Here's how the part is built. I have some questions about the finished solid (model axes, mm). A direction names the side the tool comes from. Give positions to 0.01 mm unless a question says otherwise; leave off trailing zeros. Loops run counter-clockwise (first coordinate to the right, second up) from the corner with the lowest first, then second, coordinate; pieces in that order, holes last. Notation, with made-up numbers: (61.25, 48) -> (73.25, 48) arc R24 ccw to (73.25, 74) -> close; hole circle Ø4 at (-12, 21.5). An arc over 180 degrees is marked (long way). Answer in a Markdown table with one row per item. Add a question column.
Item 1: If we section it at B-B (y = 3): Write out the boundary of the cut face in (x, z) (3 decimals), then the cut area to 3 significant figures.
Item 2: If we section it at C-C (z = 0): Give the number of separate pieces and of enclosed holes in the cut face, then the cut area to 3 significant figures.
Item 3: Which directions (+Z, -Z, +X, -X, +Y, -Y) give clear straight access to the entire face, cutting with the end or side of a thin tool? Please do faces 4 (the face through (25, 11.684, 3)), 5 (the face through (-32, 1.905, 16)), 6 (the face through (-53.84, 15.62, 25.18)).
Item 4: We'd pull the mould along Z, two halves only. Please class faces 1 (the face through (-1, 8, 28.575)), 2 (the face through (25.44, 0.94, -19.16)), 3 (the face through (-53.837, 15.625, -25.173)): released by +Z, released by -Z, zero draft, split by the parting line, or undercut.
Item 5: If we section it at D-D (z = 20): Write out the boundary of the cut face in (x, y) (3 decimals).
Item 6: If I drill on line 1 (X direction, y = 6.25, z = -1); line 2 (Z direction, x = -31.75, y = 4) (3 decimals); line 3 (X direction, y = 1.75, z = -15), over which ranges is the centre line in solid material (lowest first)?
Item 7: For P1, Ø23, axis at x = -31.75, z = -15.875, coming from the -Y side; P2, Ø5, axis at x = 28, z = 16.5, coming from the -Y side (3 decimals); P3, Ø5, axis at x = 31.75, z = 0, coming from the -Y side, each with a flat end and sliding along its axis, tell me the tip position at first contact or that it passes through.
```python
from build123d import *

# Parameters (mm, degrees)
SKETCH1_W               = 114.3
SKETCH1_H               = 57.15
EXTRUDE1_DEPTH          = 15.875
CUT_EXTRUDE1_DEPTH      = 16.875
SKETCH4_R               = 15.5575
EXTRUDE7_DEPTH          = 4.191
SKETCH6_R               = 6.858
EXTRUDE8_DEPTH          = 4.191
CHAMFER1_SIZE           = 0.508
SKETCH7_R               = 7.112
CUT_EXTRUDE2_DEPTH      = 1.905
F_1_4_20_TAPPED_HOLE1_D = 6.35


with BuildPart() as part:
    # Sketch1 → Extrude1 (new body)
    with BuildSketch(Plane(origin=(0, 0, 0), x_dir=(1, 0, 0), z_dir=(0, 1, 0))):
        Rectangle(SKETCH1_W, SKETCH1_H)
    extrude(amount=EXTRUDE1_DEPTH)

    # Sketch3 → Cut-Extrude1 (cut, through all)
    with BuildSketch(Plane(origin=(0, 15.875, 0), x_dir=(1, 0, 0), z_dir=(0, 1, 0))):
        Polygon((-57.15, 22.225), (-50.8, 28.575), (-57.15, 28.575), align=None)
        Polygon((-57.15, -28.575), (-57.15, -22.225), (-50.8, -28.575), align=None)
        Polygon((57.15, -28.575), (57.15, -22.225), (50.8, -28.575), align=None)
        Polygon((57.15, 28.575), (57.15, 22.225), (50.8, 28.575), align=None)
    extrude(amount=-CUT_EXTRUDE1_DEPTH, mode=Mode.SUBTRACT)

    # Sketch4 → Extrude7 (cut)
    with BuildSketch(Plane(origin=(0, 15.875, 0), x_dir=(1, 0, 0), z_dir=(0, 1, 0))):
        with Locations(Location((-31.75, 0, 0), (0, 0, 270))):  # turned: the seam where the file's is
            Circle(SKETCH4_R)
        with Locations(Location((31.75, 0, 0), (0, 0, 270))):  # turned: the seam where the file's is
            Circle(SKETCH4_R)
    extrude(amount=-EXTRUDE7_DEPTH, mode=Mode.SUBTRACT)

    # Sketch6 → Extrude8 (add)
    with BuildSketch(Plane(origin=(0, 11.684, 0), x_dir=(1, 0, 0), z_dir=(0, 1, 0))):
        with Locations(Location((-31.75, 0, 0), (0, 0, 270))):  # turned: the seam where the file's is
            Circle(SKETCH6_R)
        with Locations(Location((31.75, 0, 0), (0, 0, 270))):  # turned: the seam where the file's is
            Circle(SKETCH6_R)
    extrude(amount=EXTRUDE8_DEPTH)

    # Chamfer1
    chamfer1_edges = [part.edges().sort_by_distance(p)[0] for p in [
        (-57.15, 0, 0),
        (-57.15, 15.875, 0),
        (-53.975, 0, -25.4),
        (-53.975, 15.875, -25.4),
        (0, 0, 28.575),
        (0, 15.875, 28.575),
        (-53.975, 0, 25.4),
        (-53.975, 15.875, 25.4),
        (57.15, 0, 0),
        (57.15, 15.875, 0),
        (53.975, 0, 25.4),
        (53.975, 15.875, 25.4),
        (0, 0, -28.575),
        (0, 15.875, -28.575),
        (53.975, 0, -25.4),
        (53.975, 15.875, -25.4),
        (-31.75, 15.875, -15.5575),
        (31.75, 15.875, -15.5575),
        (-31.75, 15.875, -6.858),
        (31.75, 15.875, -6.858),
    ]]
    chamfer(chamfer1_edges, length=CHAMFER1_SIZE)

    # Sketch7 → Cut-Extrude2 (cut)
    with BuildSketch(Plane.XZ):
        with Locations(Location((-31.75, 15.875, 0), (0, 0, 270))):  # turned: the seam where the file's is
            Circle(SKETCH7_R)
        with Locations(Location((-31.75, -15.875, 0), (0, 0, 270))):  # turned: the seam where the file's is
            Circle(SKETCH7_R)
        with Locations(Location((31.75, 15.875, 0), (0, 0, 270))):  # turned: the seam where the file's is
            Circle(SKETCH7_R)
        with Locations(Location((31.75, -15.875, 0), (0, 0, 270))):  # turned: the seam where the file's is
            Circle(SKETCH7_R)
    extrude(amount=-CUT_EXTRUDE2_DEPTH, mode=Mode.SUBTRACT)

    # 1/4-20 Tapped Hole1 (through all)
    with Locations(Plane(origin=(0, 15.875, 0), x_dir=(-1, 0, 0), z_dir=(0, 1, 0))):
        with Locations((31.75, 0), (-31.75, 0)):
            Hole(F_1_4_20_TAPPED_HOLE1_D / 2)


solid = part.part
```
Recorded:
| question | item | result |
|---|---|---|
| 1 | outline | (-57.15, -22.225) -> (-50.8, -28.575) -> (50.8, -28.575) -> (57.15, -22.225) -> (57.15, 22.225) -> (50.8, 28.575) -> (-50.8, 28.575) -> (-57.15, 22.225) -> close; hole circle Ø6.35 at (-31.75, 0); hole circle Ø6.35 at (31.75, 0) |
| 1 | area | 6,390 mm^2 |
| 2 | separate pieces | 3 |
| 2 | enclosed holes | 0 |
| 2 | area | 1,470 mm^2 |
| 3 | face 4 | +Y |
| 3 | face 5 | -Y |
| 3 | face 6 | +Z, -X, +Y |
| 4 | face 1 | released by +Z |
| 4 | face 2 | undercut |
| 4 | face 3 | released by -Z |
| 5 | outline | (-57.15, 0.508) -> (-56.642, 0) -> (-37.544, 0) -> (-37.544, 1.905) -> (-25.956, 1.905) -> (-25.956, 0) -> (25.956, 0) -> (25.956, 1.905) -> (37.544, 1.905) -> (37.544, 0) -> (56.642, 0) -> (57.15, 0.508) -> (57.15, 15.367) -> (56.642, 15.875) -> (-56.642, 15.875) -> (-57.15, 15.367) -> close |
| 6 | line 1 | x = -57.15 to -34.76, -28.74 to 28.74, 34.76 to 57.15 |
| 6 | line 2 | z = -28.575 to -3.175, 3.175 to 28.575 |
| 6 | line 3 | x = -57.15 to -38.81, -24.69 to 24.69, 38.81 to 57.15 |
| 7 | P1 | stops at y = 0 |
| 7 | P2 | stops at y = 1.905 |
| 7 | P3 | passes through |
